```python
from build123d import *

# Parameters (mm, degrees)
F0_R     = 1.5875
F1_DEPTH = 6.35


with BuildPart() as f1:
    # F0 (on Front) → F1 (new body)
    with BuildSketch(Plane.XZ):
        Polygon((0, 25.4), (0, 0), (25.4, 0), align=None)
        with Locations((12.7, 3.175)):
            Circle(F0_R, mode=Mode.SUBTRACT)
        with Locations((3.175, 12.7)):
            Circle(F0_R, mode=Mode.SUBTRACT)
    extrude(amount=F1_DEPTH)


solid = f1.part
```
Geometry check sheet. Reference: the model listing, model coordinates, mm. Give positions to 0.01 mm unless a question says otherwise; leave off trailing zeros. Loops run counter-clockwise (first coordinate to the right, second up) from the corner with the lowest first, then second, coordinate; pieces in that order, holes last. Notation, with made-up numbers: M -39,19.25 L -34,19.25 A13 cw -34,36.25 Z; hole C 29,-7.75 d11. An arc over 180 degrees is marked long. Answer as CSV lines item,"result".
Item 1: Cross-section at A-A on x = 12.7. Record the cut outline in (y, z), and give its area (3 significant figures).
Values:
outline,"M -6.35,0 L 0,0 L 0,1.59 L -6.35,1.59 Z; M -6.35,4.76 L 0,4.76 L 0,12.7 L -6.35,12.7 Z"
area,"60.5 mm²"
Item 2: Depth check by flat-ended pin: P1, Ø1, axis at y = -4.5, z = 19, coming from the +X side; P2, Ø1.5, axis at x = 2.5, y = -4, coming from the +Z side. Enter the tip coordinate at first touch or a pass-through.
Values:
P1,"stops at x = 6.9"
P2,"stops at z = 23.65"
Item 3: Cross-section at D-D on z = 9.5. Record the cut outline in (x, y).
Values:
outline,"M 0,-6.35 L 15.9,-6.35 L 15.9,0 L 0,0 Z"
Item 4: Cross-section at C-C on y = -3.5. Record the cut outline in (x, z) (1 decimal).
Values:
outline,"M 0,0 L 25.4,0 L 0,25.4 Z; hole C 3.2,12.7 d3.2; hole C 12.7,3.2 d3.2"
Item 5: Cross-section at B-B on z = 12.7. Record the cut outline in (x, y).
Values:
outline,"M 0,-6.35 L 1.59,-6.35 L 1.59,0 L 0,0 Z; M 4.76,-6.35 L 12.7,-6.35 L 12.7,0 L 4.76,0 Z"
Item 6: Release check for a two-part mould opening along X. For faces 1 (the flat face through (12.9, -3.1, 12.5)), 2 (the cylindrical face through (2.968, -3.131, 14.274)), 3 (the flat face through (7, -6.35, 7)) record: pulls with the +X half, pulls with the -X half, needs draft (parallel to the pull), parting line crosses it, or undercut.
Values:
face 1,"pulls with the +X half"
face 2,"undercut"
face 3,"needs draft"
Item 7: Material ranges on line 1 (X direction, y = -3, z = 3.5); line 2 (Z direction, x = 24, y = -4.75); line 3 (X direction, y = -0.5, z = 11.5), recorded low to high.
Values:
line 1,"x = 0 to 11.15, 14.25 to 21.9"
line 2,"z = 0 to 1.4"
line 3,"x = 0 to 2.14, 4.21 to 13.9"
